Design review of the part built by this model. Coordinates are the model's own, in mm. Coordinates: 2 decimals unless noted, no trailing zeros. Loops run counter-clockwise (first coordinate to the right, second up) from the corner with the lowest first, then second, coordinate; pieces in that order, holes last. Notation, with made-up numbers: (-3.5, 37) -> (55.5, 37) arc R18 cw to (55.5, 63) -> close; hole circle Ø6 at (-38.5, 2). An arc over 180 degrees is marked (long way). One line per item, written item: value. Start each with the question number.
1. Add section A-A on z = 2.1. Write out the cut boundary in (x, y), plus the area to 3 significant figures.
2. Insertion check: pin 1 (10 mm diameter, centred on x = 247, y = 190, fed in from -Z); pin 2 (4 mm diameter, centred on x = 175.82, y = 326.5, fed in from -Z); pin 3 (1.5 mm diameter, centred on y = 49.5, z = 1, fed in from +X) (3 decimals). Each pin has a flat end and moves straight along its axis. Give the tip position at first contact, or say it passes through.
3. Add section C-C on y = 192. Write out the cut boundary in (x, z).
4. Add section B-B on x = 262. Write out the cut boundary in (y, z).
5. For probe 1 along X at (y, z) = (130, 1.5); probe 2 along Y at (x, z) = (277, 1.9); probe 3 along Y at (x, z) = (301, 1.45), list the stretches that pass through material, from the lowest coordinate up.
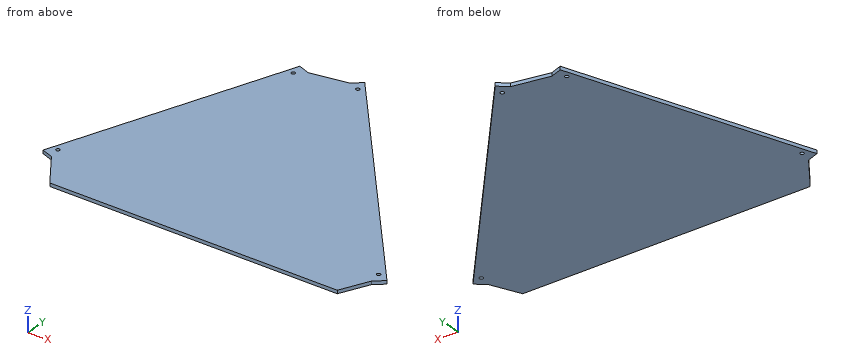
```python
from build123d import *

# Parameters (mm, degrees)
EXTRUDE_1_DEPTH    = 4
HOLE_WIZARD_M4_1_D = 4.5


with BuildPart() as part:
    # ｽｹｯﾁ1 → ﾎﾞｽ - 押し出し1 (new body)
    with BuildSketch(Plane.XY):
        Polygon((162.040656836, 331.259045811), (411.074557564, 34.47199994), (395, 0), (45, 0), (15.39090645, 42.286167935), (117.724307951, 323.444877815), align=None)
        Polygon((117.724307951, 323.444877815), (103.628918639, 328.575179965), (1.295517138, 47.416470085), (15.39090645, 42.286167935), align=None)
        Polygon((173.531323483, 340.900859956), (422.565224211, 44.113814086), (411.074557564, 34.47199994), (162.040656836, 331.259045811), align=None)
    extrude(amount=EXTRUDE_1_DEPTH)

    # M4 すきま穴1 (through all)
    with Locations(Plane.XY.offset(4)):
        with Locations((106.401361503, 314.263871131), (12.618463585, 56.59747677), (175.820835281, 326.504397344), (408.785045766, 48.868462552)):
            Hole(HOLE_WIZARD_M4_1_D / 2)


solid = part.part
```
Worked answers:
1. outline: (1.3, 47.42) -> (15.39, 42.29) -> (45, 0) -> (395, 0) -> (411.07, 34.47) -> (422.57, 44.11) -> (173.53, 340.9) -> (162.04, 331.26) -> (117.72, 323.44) -> (103.63, 328.58) -> close; hole circle Ø4.5 at (12.62, 56.6); hole circle Ø4.5 at (106.4, 314.26); hole circle Ø4.5 at (175.82, 326.5); hole circle Ø4.5 at (408.79, 48.87)
1. area: 88,100 mm²
2. pin 1: stops at z = 0
2. pin 2: passes through
2. pin 3: stops at x = 418.675
3. outline: (53.92, 0) -> (298.47, 0) -> (298.47, 4) -> (53.92, 4) -> close
4. outline: (0, 0) -> (235.47, 0) -> (235.47, 4) -> (0, 4) -> close
5. probe 1: x = 31.35 to 350.5
5. probe 2: y = 0 to 217.59
5. probe 3: y = 0 to 188.99
